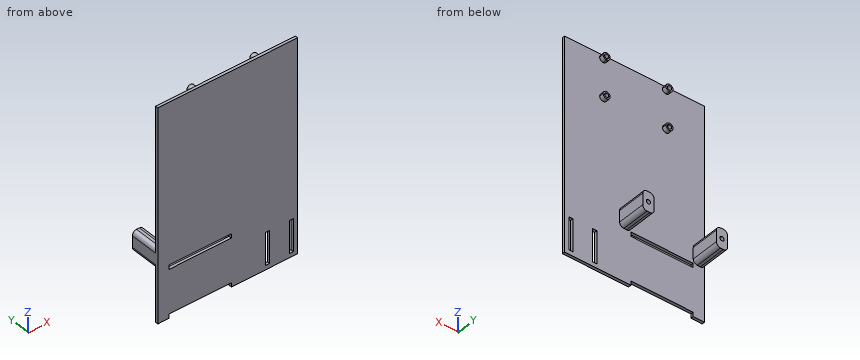
```python
from build123d import *

# Parameters (mm, degrees)
SKETCH1_W           = 99
SKETCH1_H           = 150
BOSS_EXTRUDE1_DEPTH = 2
SKETCH2_W           = 8
SKETCH2_H           = 14
BOSS_EXTRUDE2_DEPTH = 20
SKETCH3_R           = 1.5
CUT_EXTRUDE2_DEPTH  = 15
FILLET1_R           = 3
FILLET2_R           = 3
FILLET5_R           = 3
FILLET6_R           = 3
FILLET7_R           = 3
FILLET8_R           = 3
FILLET9_R           = 3
FILLET10_R          = 3
SKETCH5_W           = 44.075
SKETCH5_H           = 3
SKETCH5_W_2         = 2.852474079
SKETCH5_H_2         = 23
SKETCH5_W_3         = 3
CUT_EXTRUDE3_DEPTH  = 10
BOSS_EXTRUDE3_DEPTH = 3


with BuildPart() as part:
    # Sketch1 → Boss-Extrude1 (new body)
    with BuildSketch(Plane(origin=(0, 0, 0), x_dir=(1, 0, 0), z_dir=(0, 1, 0))):
        with Locations((49.5, 75)):
            Rectangle(SKETCH1_W, SKETCH1_H)
    extrude(amount=BOSS_EXTRUDE1_DEPTH)

    # Sketch2 → Boss-Extrude2 (add)
    with BuildSketch(Plane(origin=(0, 2, 0), x_dir=(1, 0, 0), z_dir=(0, 1, 0))):
        with Locations((4, 106)):
            Rectangle(SKETCH2_W, SKETCH2_H)
        with Locations((56.075, 106)):
            Rectangle(SKETCH2_W, SKETCH2_H)
    extrude(amount=BOSS_EXTRUDE2_DEPTH)

    # Sketch3 → Cut-Extrude2 (cut)
    with BuildSketch(Plane(origin=(0, 22, 0), x_dir=(1, 0, 0), z_dir=(0, 1, 0))):
        with Locations((56.075, 106)):
            Circle(SKETCH3_R)
        with Locations((4, 106)):
            Circle(SKETCH3_R)
    extrude(amount=-CUT_EXTRUDE2_DEPTH, mode=Mode.SUBTRACT)

    # Fillet1
    fillet1_edges = [part.edges().sort_by_distance(p)[0] for p in [
        (0, 12, -99),
    ]]
    fillet(fillet1_edges, radius=FILLET1_R)

    # Fillet2
    fillet2_edges = [part.edges().sort_by_distance(p)[0] for p in [
        (0, 12, -113),
    ]]
    fillet(fillet2_edges, radius=FILLET2_R)

    # Fillet5
    fillet5_edges = [part.edges().sort_by_distance(p)[0] for p in [
        (8, 12, -113),
    ]]
    fillet(fillet5_edges, radius=FILLET5_R)

    # Fillet6
    fillet6_edges = [part.edges().sort_by_distance(p)[0] for p in [
        (8, 12, -99),
    ]]
    fillet(fillet6_edges, radius=FILLET6_R)

    # Fillet7
    fillet7_edges = [part.edges().sort_by_distance(p)[0] for p in [
        (60.075, 12, -99),
    ]]
    fillet(fillet7_edges, radius=FILLET7_R)

    # Fillet8
    fillet8_edges = [part.edges().sort_by_distance(p)[0] for p in [
        (60.075, 12, -113),
    ]]
    fillet(fillet8_edges, radius=FILLET8_R)

    # Fillet9
    fillet9_edges = [part.edges().sort_by_distance(p)[0] for p in [
        (52.075, 12, -113),
    ]]
    fillet(fillet9_edges, radius=FILLET9_R)

    # Fillet10
    fillet10_edges = [part.edges().sort_by_distance(p)[0] for p in [
        (52.075, 12, -99),
    ]]
    fillet(fillet10_edges, radius=FILLET10_R)

    # Sketch5 → Cut-Extrude3 (cut)
    with BuildSketch(Plane(origin=(0, 2, 0), x_dir=(1, 0, 0), z_dir=(0, 1, 0))):
        with Locations((30.0375, 148.5)):
            Rectangle(SKETCH5_W, SKETCH5_H)
        with Locations((30.0375, 114.5)):
            Rectangle(SKETCH5_W, SKETCH5_H)
        with Locations((94.573762961, 135.5)):
            Rectangle(SKETCH5_W_2, SKETCH5_H_2)
        with Locations((77.647525921, 135.5)):
            Rectangle(SKETCH5_W_3, SKETCH5_H_2)
    extrude(amount=-CUT_EXTRUDE3_DEPTH, mode=Mode.SUBTRACT)

    # Sketch6 → Boss-Extrude3 (add)
    with BuildSketch(Plane(origin=(0, 2, 0), x_dir=(1, 0, 0), z_dir=(0, 1, 0))):
        with BuildLine():
            ThreePointArc((29.79, 29.5), (25.522233047, 31.267766953), (27.29, 27))
            Line((27.29, 27), (27.29, 28))
            ThreePointArc((27.29, 28), (26.229339828, 30.560660172), (28.79, 29.5))
            Line((28.79, 29.5), (29.79, 29.5))
        make_face()
        with BuildLine():
            Line((27.29, 28), (27.29, 27))
            ThreePointArc((27.29, 27), (29.057766953, 27.732233047), (29.79, 29.5))
            Line((29.79, 29.5), (28.79, 29.5))
            ThreePointArc((28.79, 29.5), (28.350660172, 28.439339828), (27.29, 28))
        make_face()
        with BuildLine():
            ThreePointArc((69.21, 29.5), (69.942233047, 27.732233047), (71.71, 27))
            Line((71.71, 27), (71.71, 28))
            ThreePointArc((71.71, 28), (70.649339828, 28.439339828), (70.21, 29.5))
            Line((70.21, 29.5), (69.21, 29.5))
        make_face()
        with BuildLine():
            Line((71.71, 28), (71.71, 27))
            ThreePointArc((71.71, 27), (73.477766953, 27.732233047), (74.21, 29.5))
            ThreePointArc((74.21, 29.5), (71.71, 32), (69.21, 29.5))
            Line((69.21, 29.5), (70.21, 29.5))
            ThreePointArc((70.21, 29.5), (71.71, 31), (73.21, 29.5))
            ThreePointArc((73.21, 29.5), (72.770660172, 28.439339828), (71.71, 28))
        make_face()
        with BuildLine():
            ThreePointArc((27.29, 5), (25.522233047, 0.732233047), (29.79, 2.5))
            Line((29.79, 2.5), (28.79, 2.5))
            ThreePointArc((28.79, 2.5), (26.229339828, 1.439339828), (27.29, 4))
            Line((27.29, 4), (27.29, 5))
        make_face()
        with BuildLine():
            Line((28.79, 2.5), (29.79, 2.5))
            ThreePointArc((29.79, 2.5), (29.057766953, 4.267766953), (27.29, 5))
            Line((27.29, 5), (27.29, 4))
            ThreePointArc((27.29, 4), (28.350660172, 3.560660172), (28.79, 2.5))
        make_face()
        with BuildLine():
            ThreePointArc((71.71, 5), (69.942233047, 4.267766953), (69.21, 2.5))
            Line((69.21, 2.5), (70.21, 2.5))
            ThreePointArc((70.21, 2.5), (70.649339828, 3.560660172), (71.71, 4))
            Line((71.71, 4), (71.71, 5))
        make_face()
        with BuildLine():
            Line((70.21, 2.5), (69.21, 2.5))
            ThreePointArc((69.21, 2.5), (71.71, 0), (74.21, 2.5))
            ThreePointArc((74.21, 2.5), (73.477766953, 4.267766953), (71.71, 5))
            Line((71.71, 5), (71.71, 4))
            ThreePointArc((71.71, 4), (72.770660172, 3.560660172), (73.21, 2.5))
            ThreePointArc((73.21, 2.5), (71.71, 1), (70.21, 2.5))
        make_face()
    extrude(amount=BOSS_EXTRUDE3_DEPTH)


solid = part.part
```
Here's how the part is built. I have some questions about the finished solid (model axes, mm). Round coordinates to 2 decimals unless told otherwise and drop trailing zeros. Write each loop counter-clockwise with the first axis right and the second up, starting at its lowest first coordinate (ties: lowest second). Pieces come first, ordered by that corner, then holes. Notation, with made-up numbers: M -32,-20.5 L 27,-20.5 A20 cw 27,-2.5 Z; hole C 79.5,38 d2. An arc over 180 degrees is marked long. Answer as CSV lines item,"result". Start each with the question number.
1. Suppose I cut it at B-B on z = -106. Write out the boundary of the cut face in (x, y) (3 decimals).
2. I'm going to push flat-ended pins straight in: pin 1 Ø4 at (x, z) = (34, -57) entering from +Y; pin 2 Ø1.6 at (x, y) = (4, 11.5) entering from +Z; pin 3 Ø2.5 at (x, z) = (27.5, -1.5) entering from +Y; pin 4 Ø5 at (y, z) = (5, -18) entering from +X. Where does each tip first touch, or does it pass through?
3. I need wall thicknesses on probe 1 along X at (y, z) = (3.85, -29.5); probe 2 along X at (y, z) = (11.75, -106) (3 decimals); probe 3 along Z at (x, y) = (56, 8.25). Which ranges of each line are inside material? Lowest first, please.
4. Suppose I cut it at A-A on y = 11.5. Write out the boundary of the cut face in (x, z) (3 decimals), then the cut area to 3 significant figures.
5. Suppose I cut it at C-C on x = 64. Write out the boundary of the cut face in (y, z), then the cut area to 3 significant figures.
6. Suppose I cut it at D-D on z = -45. Write out the boundary of the cut face in (x, y), then the cut area to 3 significant figures.
Check result:
1,outline,"M 0,0 L 99,0 L 99,2 L 60.075,2 L 60.075,22 L 57.575,22 L 57.575,7 L 54.575,7 L 54.575,22 L 52.075,22 L 52.075,2 L 8,2 L 8,22 L 5.5,22 L 5.5,7 L 2.5,7 L 2.5,22 L 0,22 Z"
2,pin 1,"stops at y = 2"
2,pin 2,"stops at z = -99"
2,pin 3,"stops at y = 5"
2,pin 4,"passes through"
3,probe 1,"x = 24.79 to 25.79, 28.79 to 29.79, 69.21 to 70.21, 73.21 to 74.21"
3,probe 2,"x = 0 to 2.5, 5.5 to 8, 52.075 to 54.575, 57.575 to 60.075"
3,probe 3,"z = -113 to -107.5, -104.5 to -99"
4,outline,"M 0,-110 A3 ccw 3,-113 L 5,-113 A3 ccw 8,-110 L 8,-102 A3 ccw 5,-99 L 3,-99 A3 ccw 0,-102 Z; M 52.075,-110 A3 ccw 55.075,-113 L 57.075,-113 A3 ccw 60.075,-110 L 60.075,-102 A3 ccw 57.075,-99 L 55.075,-99 A3 ccw 52.075,-102 Z; hole C 4,-106 d3; hole C 56.075,-106 d3"
4,area,"194 mm2"
5,outline,"M 0,-150 L 2,-150 L 2,0 L 0,0 Z"
5,area,"300 mm2"
6,outline,"M 0,0 L 99,0 L 99,2 L 0,2 Z"
6,area,"198 mm2"
